Can you work these out from the drawing? Everything is in mm from the part's minimum corner. A direction names the side the tool comes from. Round coordinates to 2 decimals unless told otherwise and drop trailing zeros. Write each loop counter-clockwise with the first axis right and the second up, starting at its lowest first coordinate (ties: lowest second). Pieces come first, ordered by that corner, then holes. Notation, with made-up numbers: (35, -22) -> (66, -22) arc R26 cw to (66, 0) -> close; hole circle Ø11 at (72, 59.5). An arc over 180 degrees is marked (long way). Answer as CSV lines item,"result". Start each with the question number.
Q1. Imagine slicing it at D-D on x = 42.5. Please give me the cut outline in (y, z).
Q2. Imagine slicing it at B-B on x = 5. Please give me the cut outline in (y, z).
Q3. If we mould it in two halves opening along Z, with no side actions, what happens to the marked faces 1, 2, 3 and 4? For each: pulls with the +Z half, pulls with the -Z half, needs draft (parallel to the pull), parting line crosses it, or undercut.
Q4. If I drill on line 1 (Z direction, x = 42, y = 4) (1 decimal); line 2 (Z direction, x = 42, y = 32); line 3 (X direction, y = 9, z = 42.5), over which ranges is the centre line in solid material (lowest first)? Write a range as [from, to].
Q5. For the marked faces 5 and 6, which set-ups out of +Z, -Z, +X, -X, +Y, -Y let a thin tool reach every point of the face, with its end or its side?
Q6. Will these pins go through, and if not, where does the flat tip stop? pin 1 Ø2 at (x, z) = (80, 42.5) entering from -Y; pin 2 Ø5.5 at (x, z) = (15.98, 69.02) entering from -Y; pin 3 Ø5 at (y, z) = (4, 64) entering from +X (1 decimal); pin 4 Ø2 at (y, z) = (13.5, 69) entering from -X.
Q7. Imagine slicing it at C-C on z = 5. Please give me the cut outline in (x, y).
Q8. Imagine slicing it at A-A on z = 42.5. Please give me the cut outline in (x, y).
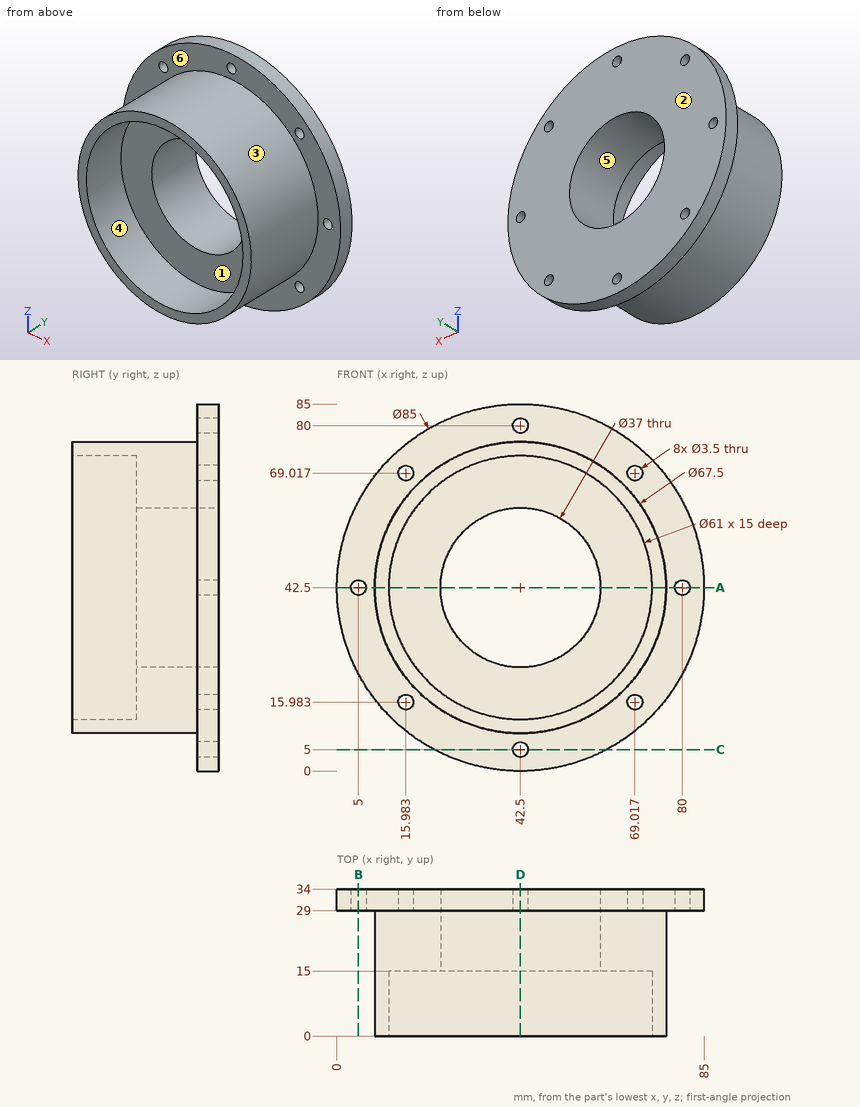
Checks:
1,outline,"(0, 8.75) -> (29, 8.75) -> (29, 6.75) -> (34, 6.75) -> (34, 24) -> (15, 24) -> (15, 12) -> (0, 12) -> close; (0, 73) -> (15, 73) -> (15, 61) -> (34, 61) -> (34, 78.25) -> (29, 78.25) -> (29, 76.25) -> (0, 76.25) -> close; (29, 0) -> (34, 0) -> (34, 3.25) -> (29, 3.25) -> close; (29, 81.75) -> (34, 81.75) -> (34, 85) -> (29, 85) -> close"
2,outline,"(29, 22.5) -> (34, 22.5) -> (34, 40.75) -> (29, 40.75) -> close; (29, 44.25) -> (34, 44.25) -> (34, 62.5) -> (29, 62.5) -> close"
3,face 1,"undercut"
3,face 2,"needs draft"
3,face 3,"parting line crosses it"
3,face 4,"undercut"
4,line 1,"[8.8, 12], [73, 76.2]"
4,line 2,"[0, 3.32], [6.68, 24.01], [60.99, 78.32], [81.68, 85]"
4,line 3,"[8.75, 12], [73, 76.25]"
5,face 5,"+Y, -Y"
5,face 6,"-Y"
6,pin 1,"through"
6,pin 2,"y = 29"
6,pin 3,"x = 70.4"
6,pin 4,"x = 20.39"
7,outline,"(22.5, 29) -> (40.75, 29) -> (40.75, 34) -> (22.5, 34) -> close; (44.25, 29) -> (62.5, 29) -> (62.5, 34) -> (44.25, 34) -> close"
8,outline,"(0, 29) -> (3.25, 29) -> (3.25, 34) -> (0, 34) -> close; (6.75, 29) -> (8.75, 29) -> (8.75, 0) -> (12, 0) -> (12, 15) -> (24, 15) -> (24, 34) -> (6.75, 34) -> close; (61, 15) -> (73, 15) -> (73, 0) -> (76.25, 0) -> (76.25, 29) -> (78.25, 29) -> (78.25, 34) -> (61, 34) -> close; (81.75, 29) -> (85, 29) -> (85, 34) -> (81.75, 34) -> close"
